Could you check a few things on this model? Use its own coordinates, in mm. A direction names the side the tool comes from. Give positions to 0.01 mm unless a question says otherwise; leave off trailing zeros. Order: outer loops, then holes, each group sorted by start corner. A loop starts at its lowest first (then second) coordinate and runs counter-clockwise, first axis right, second up. Notation, with made-up numbers: M 54,28 L 105,28 A15 ccw 105,46 Z; hole C 64.25,56 d1. An arc over 180 degrees is marked long. Return JSON: item names as keys, results as strings. Group by question number.
```python
from build123d import *

# Parameters (mm, degrees)
TOP_DEPTH                 = 2.54
SKETCH7_R                 = 1.905
BUTTONLEDCUT_DEPTH        = 72.306909304
SKETCH8_W                 = 33.528
SKETCH8_H                 = 36.195
SOLARCUT_DEPTH            = 72.306909304
F_6_32_TAPPED_HOLE1_D     = 2.7051
F_6_32_TAPPED_HOLE1_DEPTH = 11.176
F_6_32_TAPPED_HOLE1_TIP   = 0.81269403
SKETCH13_W                = 12.446
SKETCH13_H                = 1.27
BODY_TABS_DEPTH           = 1.27
BODY_TABS_DRAFT           = 7
BODY_TABS_PROFILE_2_DEPTH = 1.27
BODY_TABS_PROFILE_2_DRAFT = 7
SKETCH14_W                = 6.985
SKETCH14_H                = 1.905
FLAT_HEAD_HOLE_DEPTH      = 73.383371188


with BuildPart() as part:
    # Sketch2 → top (new body)
    with BuildSketch(Plane(origin=(0, 0, 0), x_dir=(1, 0, 0), z_dir=(0, 1, 0))):
        with BuildLine():
            Line((-25.3365, -60.2615), (25.3365, -60.2615))
            ThreePointArc((25.3365, -60.2615), (34.316756121, -56.541756121), (38.0365, -47.5615))
            Line((38.0365, -47.5615), (38.0365, 47.5615))
            ThreePointArc((38.0365, 47.5615), (34.316756121, 56.541756121), (25.3365, 60.2615))
            Line((25.3365, 60.2615), (-25.3365, 60.2615))
            ThreePointArc((-25.3365, 60.2615), (-34.316756121, 56.541756121), (-38.0365, 47.5615))
            Line((-38.0365, 47.5615), (-38.0365, -47.5615))
            ThreePointArc((-38.0365, -47.5615), (-34.316756121, -56.541756121), (-25.3365, -60.2615))
        make_face()
    extrude(amount=TOP_DEPTH)

    # Sketch7 → ButtonLEDCut (cut, through all)
    with BuildSketch(Plane(origin=(0, 2.54, 0), x_dir=(1, 0, 0), z_dir=(0, 1, 0))):
        with Locations(Location((1.3335, -51.3715, 0), (0, 0, 270))):
            Circle(SKETCH7_R)
        with Locations(Location((8.9535, -51.3715, 0), (0, 0, 270))):
            Circle(SKETCH7_R)
        with Locations(Location((8.9535, -42.4815, 0), (0, 0, 270))):
            Circle(SKETCH7_R)
        with Locations(Location((1.3335, -42.4815, 0), (0, 0, 270))):
            Circle(SKETCH7_R)
        with BuildLine():
            Line((16.8275, -46.2915), (16.8275, -47.5615))
            ThreePointArc((16.8275, -47.5615), (15.5575, -48.8315), (14.2875, -47.5615))
            Line((14.2875, -47.5615), (14.2875, -46.2915))
            ThreePointArc((14.2875, -46.2915), (15.5575, -45.0215), (16.8275, -46.2915))
        make_face()
    extrude(amount=-BUTTONLEDCUT_DEPTH, mode=Mode.SUBTRACT)

    # Sketch8 → SolarCut (cut, through all)
    with BuildSketch(Plane(origin=(0, 2.54, 0), x_dir=(1, 0, 0), z_dir=(0, 1, 0))):
        with Locations((0, 38.354)):
            Rectangle(SKETCH8_W, SKETCH8_H)
    extrude(amount=-SOLARCUT_DEPTH, mode=Mode.SUBTRACT)

    # #6-32 Tapped Hole1
    with Locations(Plane(origin=(0, 2.54, 0), x_dir=(1, 0, 0), z_dir=(0, 1, 0))):
        with Locations((-15.8115, 3.2385), (19.1135, 3.2385), (19.1135, -53.9115), (-15.8115, -53.9115)):
            Hole(F_6_32_TAPPED_HOLE1_D / 2, depth=F_6_32_TAPPED_HOLE1_DEPTH)
            with Locations((0, 0, -(F_6_32_TAPPED_HOLE1_DEPTH + F_6_32_TAPPED_HOLE1_TIP / 2))):  # 118° drill point
                Cone(0, F_6_32_TAPPED_HOLE1_D / 2, F_6_32_TAPPED_HOLE1_TIP, mode=Mode.SUBTRACT)


with BuildPart() as body_tabs_tool:
    # Sketch13 → Body Tabs (with draft: the straight prism first)
    with BuildSketch(Plane(origin=(0, 0, -60.2615), x_dir=(-1, 0, 0), z_dir=(0, 0, -1))):
        with Locations((-12.7, 0.635)):
            Rectangle(SKETCH13_W, SKETCH13_H)
    extrude(amount=BODY_TABS_DEPTH)
    # Body Tabs: the draft: its side faces are tilted about the plane it starts from
    body_tabs_sides = [body_tabs_tool.faces().sort_by_distance(p)[0] for p in [
        (12.7, 0, -60.8965),
        (6.477, 0.635, -60.8965),
        (12.7, 1.27, -60.8965),
        (18.923, 0.635, -60.8965),
    ]]
    draft(body_tabs_sides, Plane(origin=(0, 0, -60.2615), x_dir=(-1, 0, 0), z_dir=(0, 0, -1)), BODY_TABS_DRAFT)


with BuildPart() as part_1:
    add(part.part)

    # Body Tabs: add body_tabs_tool
    add(body_tabs_tool.part)


with BuildPart() as body_tabs_profile_2_tool:
    # Sketch13 → Body Tabs profile 2 (with draft: the straight prism first)
    with BuildSketch(Plane(origin=(0, 0, -60.2615), x_dir=(-1, 0, 0), z_dir=(0, 0, -1))):
        with Locations((12.7, 0.635)):
            Rectangle(SKETCH13_W, SKETCH13_H)
    extrude(amount=BODY_TABS_PROFILE_2_DEPTH)
    # Body Tabs profile 2: the draft: its side faces are tilted about the plane it starts from
    body_tabs_profile_2_sides = [body_tabs_profile_2_tool.faces().sort_by_distance(p)[0] for p in [
        (-18.923, 0.635, -60.8965),
        (-12.7, 1.27, -60.8965),
        (-6.477, 0.635, -60.8965),
        (-12.7, 0, -60.8965),
    ]]
    draft(body_tabs_profile_2_sides, Plane(origin=(0, 0, -60.2615), x_dir=(-1, 0, 0), z_dir=(0, 0, -1)), BODY_TABS_PROFILE_2_DRAFT)


with BuildPart() as part_2:
    add(part_1.part)

    # Body Tabs profile 2: add body_tabs_profile_2_tool
    add(body_tabs_profile_2_tool.part)

    # Sketch14 → Flat Head Hole (cut, through all)
    with BuildSketch(Plane(origin=(0, 2.54, 0), x_dir=(1, 0, 0), z_dir=(0, 1, 0))):
        with Locations((0, -59.309)):
            Rectangle(SKETCH14_W, SKETCH14_H)
    extrude(amount=-FLAT_HEAD_HOLE_DEPTH, mode=Mode.SUBTRACT)


solid = part_2.part
```
1. Imagine slicing it at C-C, the plane y = 1.75. Count the separate pieces of the cut face and the enclosed holes in it, plus the area to 3 significant figures.
2. I need wall thicknesses on L1, parallel to Z at x = 19.5, y = 2.4; L2, parallel to X at y = 0.9, z = -3; L3, parallel to X at y = 0.65, z = -37. Which ranges of each line are inside material? Lowest first, please. Write a range as from..to.
3. Imagine slicing it at B-B, the plane x = -10.5. Please give me the cut outline in (y, z), plus the area to 3 significant figures.
4. For pin 1 (1 mm diameter, centred on x = 26.5, y = 2, fed in from +Z); pin 2 (4.5 mm diameter, centred on x = -15.81, z = -3.24, fed in from -Y), each with a flat end and sliding along its axis, tell me the tip position at first contact or that it passes through.
5. If we mould it in two halves opening along X, with no side actions, what happens to faces 5 (the cylindrical face through (-34.22, 1.25, -56.64)), 6 (the flat face through (0, 1, -56.451)), 7 (the cylindrical face through (34.415, 1.252, -56.442))? For each: pulls with the +X half, pulls with the -X half, needs draft (parallel to the pull), parting line crosses it, or undercut.
6. Imagine slicing it at A-A, the plane z = -30. Please give me the cut outline in (x, y), plus the area to 3 significant figures.
7. Which directions (+Z, -Z, +X, -X, +Y, -Y) give clear straight access to the entire face, cutting with the end or side of a thin tool? Please do faces 1 (the flat face through (16.764, 1, -38)), 2 (the flat face through (0, 2, -60.262)), 3 (the flat face through (-15, 1, 60.262)), 4 (the flat face through (0, 1, 58.356)).
Values:
{
 "1": {"separate pieces": "1", "enclosed holes": "10", "area": "7,730 mm²"},
 "2": {"L1": "z = -60.26..-4.53, -1.94..52.62, 55.21..60.26", "L2": "x = -38.04..-17.14, -14.48..17.78, 20.44..38.04", "L3": "x = -38.04..-16.76, 16.76..38.04"},
 "3": {"outline": "M 0,-60.26 L 0.16,-61.53 L 1.11,-61.53 L 1.27,-60.26 L 2.54,-60.26 L 2.54,-56.45 L 0,-56.45 Z; M 0,-20.26 L 2.54,-20.26 L 2.54,60.26 L 0,60.26 Z", "area": "216 mm²"},
 "4": {"pin 1": "stops at z = 60.24", "pin 2": "stops at y = 0"},
 "5": {"face 5": "pulls with the -X half", "face 6": "undercut", "face 7": "pulls with the +X half"},
 "6": {"outline": "M -38.04,0 L -16.76,0 L -16.76,2.54 L -38.04,2.54 Z; M 16.76,0 L 38.04,0 L 38.04,2.54 L 16.76,2.54 Z", "area": "108 mm²"},
 "7": {"face 1": "+Y, -Y", "face 2": "-Z, +Y", "face 3": "+Z, +X, -X, +Y, -Y", "face 4": "+Z, +Y, -Y"}
}
